Geometry check sheet. Reference: the model listing, model coordinates, mm. Coordinates: 2 decimals unless noted, no trailing zeros. Order: outer loops, then holes, each group sorted by start corner. A loop starts at its lowest first (then second) coordinate and runs counter-clockwise, first axis right, second up. Notation, with made-up numbers: (53.5, 20) - (107.5, 20) arc R33 ccw to (107.5, 54) - close; hole circle Ø3 at (86.25, 56). An arc over 180 degrees is marked (long way). Use CSV: the item, a comma, the result in double quotes. Start each with the question number.
1) Sectioned sample at A-A, the plane z = -10.5. Record the cut outline in (x, y), and give its area (3 significant figures).
2) Sectioned sample at B-B, the plane x = 0. Record the cut outline in (y, z), and give its area (3 significant figures).
3) Draft check along Z on faces 1 (the flat face through (0, 45, -14.5)), 2 (the cylindrical face through (0.14, 43.588, -10.236)), 3 (the flat face through (0, 45, 11.5)), 4 (the flat face through (10, 45, -1)). Enter one of: released by +Z, released by -Z, zero draft, split by the parting line, or undercut.
4) Sectioned sample at C-C, the plane y = 45.25. Record the cut outline in (x, z).
5) Depth check by flat-ended pin: P1, Ø2.5, axis at x = 0, z = 7.5, coming from the +Y side; P2, Ø5, axis at x = -0.5, z = 1, coming from the -Y side. Enter the tip coordinate at first touch or a pass-through.
6) Sectioned sample at D-D, the plane x = -5. Record the cut outline in (y, z).
7) Thickness scan on probe 1 along X at (y, z) = (41.25, -7.5); probe 2 along Z at (x, y) = (0, 44.5); probe 3 along Z at (x, y) = (-5.75, 44.5). Record the ranges inside material, lowest first. Write a range as [from, to].
from build123d import *

# Parameters (mm, degrees)
BOSS_EXTRUDE1_DEPTH             = 11.5
F_2_56_TAPPED_HOLE3_D           = 1.778
F_2_56_TAPPED_HOLE3_CSINK_D     = 3.4544
F_2_56_TAPPED_HOLE3_CSINK_ANGLE = 90
BOSS_EXTRUDE2_DEPTH             = 3
F_2_CLEARANCE_HOLE1_D           = 2.4384


with BuildPart() as part:
    # Sketch1 → Boss-Extrude1 (new body, symmetric)
    with BuildSketch(Plane.XY):
        with BuildLine():
            Line((-10, 39.778288752), (-10, 49.778288752))
            Line((-10, 49.778288752), (10, 49.778288752))
            Line((10, 49.778288752), (10, 39.778288752))
            ThreePointArc((10, 39.778288752), (0, 41.016), (-10, 39.778288752))
        make_face()
    extrude(amount=BOSS_EXTRUDE1_DEPTH, both=True)

    # #2-56 Tapped Hole3 (through all)
    with Locations(Plane(origin=(0, 49.778288752, 0), x_dir=(1, 0, 0), z_dir=(0, 1, 0))):
        with Locations((0, -7.5), (0, 7.5)):
            CounterSinkHole(F_2_56_TAPPED_HOLE3_D / 2, F_2_56_TAPPED_HOLE3_CSINK_D / 2, counter_sink_angle=F_2_56_TAPPED_HOLE3_CSINK_ANGLE)

    # Sketch5 → Boss-Extrude2 (add)
    with BuildSketch(Plane(origin=(0, 0, -11.5), x_dir=(-1, 0, 0), z_dir=(0, 0, -1))):
        with BuildLine():
            Line((10, 49.778288752), (-10, 49.778288752))
            Line((-10, 49.778288752), (-10, 39.778288752))
            ThreePointArc((-10, 39.778288752), (0, 41.016), (10, 39.778288752))
            Line((10, 39.778288752), (10, 49.778288752))
        make_face()
    extrude(amount=BOSS_EXTRUDE2_DEPTH)

    # #2 Clearance Hole1 (through all)
    with Locations(Plane.ZY.offset(10)):
        with Locations((-10.5, 44.778288752)):
            Hole(F_2_CLEARANCE_HOLE1_D / 2)


solid = part.part
Evaluation:
1,outline,"(-10, 39.78) arc R41.02 cw to (10, 39.78) - (10, 43.56) - (-10, 43.56) - close; (-10, 46) - (10, 46) - (10, 49.78) - (-10, 49.78) - close"
1,area,"135 mm²"
2,outline,"(41.02, -14.5) - (49.78, -14.5) - (49.78, -9.23) - (48.94, -8.39) - (41.02, -8.39) - close; (41.02, -6.61) - (48.94, -6.61) - (49.78, -5.77) - (49.78, 5.77) - (48.94, 6.61) - (41.02, 6.61) - close; (41.02, 8.39) - (48.94, 8.39) - (49.78, 9.23) - (49.78, 11.5) - (41.02, 11.5) - close; hole circle Ø2.44 at (44.78, -10.5)"
2,area,"191 mm²"
3,face 1,"released by -Z"
3,face 2,"undercut"
3,face 3,"released by +Z"
3,face 4,"zero draft"
4,outline,"(-10, -14.5) - (10, -14.5) - (10, -11.62) - (-10, -11.62) - close; (-10, -9.38) - (10, -9.38) - (10, 11.5) - (-10, 11.5) - close; hole circle Ø1.78 at (0, -7.5); hole circle Ø1.78 at (0, 7.5)"
5,P1,"y = 49.3"
5,P2,"y = 40.91"
6,outline,"(40.71, -14.5) - (49.78, -14.5) - (49.78, 11.5) - (40.71, 11.5) - close; hole circle Ø2.44 at (44.78, -10.5)"
7,probe 1,"[-10, -0.89], [0.89, 10]"
7,probe 2,"[-14.5, -11.69], [-9.31, -8.39], [-6.61, 6.61], [8.39, 11.5]"
7,probe 3,"[-14.5, -11.69], [-9.31, 11.5]"
